Can you work these out from the drawing? Everything is in mm from the part's minimum corner. Round coordinates to 2 decimals unless told otherwise and drop trailing zeros. Loops run counter-clockwise (first coordinate to the right, second up) from the corner with the lowest first, then second, coordinate; pieces in that order, holes last. Notation, with made-up numbers: (-6.75, -4) -> (41.25, -4) arc R31 ccw to (41.25, 33) -> close; hole circle Ø2 at (54, 73). An arc over 180 degrees is marked (long way). One line per item, written item: value.
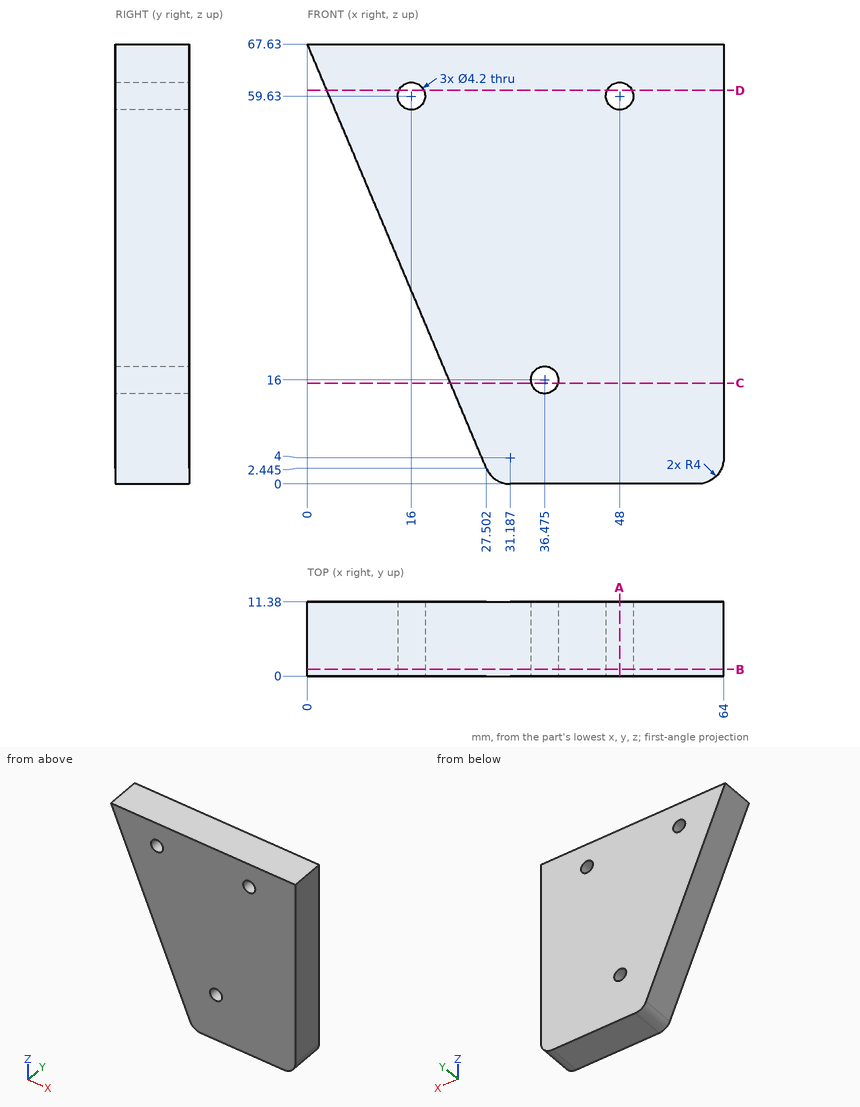
(1) If we section it at B-B, the plane y = 1: Please give me the cut outline in (x, z) (1 decimal).
Recorded:
outline: (0, 67.6) -> (27.5, 2.4) arc R4 ccw to (31.2, 0) -> (60, 0) arc R4 ccw to (64, 4) -> (64, 67.6) -> close; hole circle Ø4.2 at (16, 59.6); hole circle Ø4.2 at (36.5, 16); hole circle Ø4.2 at (48, 59.6)
(2) I'm going to push flat-ended pins straight in: pin 1 Ø1.5 at (x, y) = (25.5, 10) entering from -Z (1 decimal); pin 2 Ø4 at (y, z) = (2, 35) entering from -X. Where does each tip first touch, or does it pass through?
Recorded:
pin 1: z = 5.4
pin 2: x = 12.92
(3) If we section it at A-A, the plane x = 48: Please give me the cut outline in (y, z).
Recorded:
outline: (0, 0) -> (11.38, 0) -> (11.38, 57.53) -> (0, 57.53) -> close; (0, 61.73) -> (11.38, 61.73) -> (11.38, 67.63) -> (0, 67.63) -> close
(4) If we section it at D-D, the plane z = 60.5: Please give me the cut outline in (x, y).
Recorded:
outline: (3.01, 0) -> (14.09, 0) -> (14.09, 11.38) -> (3.01, 11.38) -> close; (17.91, 0) -> (46.09, 0) -> (46.09, 11.38) -> (17.91, 11.38) -> close; (49.91, 0) -> (64, 0) -> (64, 11.38) -> (49.91, 11.38) -> close
(5) If I drill on L1, parallel to X at y = 5, z = 59.63 (1 decimal); L2, parallel to Z at x = 37, y = 2; L3, parallel to Z at x = 49.5, y = 5, over which ranges is the centre line in solid material (lowest first)?
Recorded:
L1: 3.4 to 13.9, 18.1 to 45.9, 50.1 to 64
L2: 0 to 13.97, 18.03 to 67.63
L3: 0 to 58.16, 61.1 to 67.63
(6) If we section it at C-C, the plane z = 15.5: Please give me the cut outline in (x, y) (1 decimal), then the cut area to 3 significant figures.
Recorded:
outline: (22, 0) -> (34.4, 0) -> (34.4, 11.4) -> (22, 11.4) -> close; (38.5, 0) -> (64, 0) -> (64, 11.4) -> (38.5, 11.4) -> close
area: 432 mm²
